Geometry: final body of the model. Coordinates: model frame, mm. Round coordinates to 2 decimals unless told otherwise and drop trailing zeros. Loops run counter-clockwise (first coordinate to the right, second up) from the corner with the lowest first, then second, coordinate; pieces in that order, holes last. Notation, with made-up numbers: (10, -33.75) - (58, -33.75) arc R24 ccw to (58, -8.75) - close; hole circle Ø9 at (11, 2). An arc over 180 degrees is marked (long way). Return JSON: item names as keys, results as strings. Group by question number.
1. Section C-C on y = -11. Return loops of the section in (x, z).
2. Section B-B on y = -6.75. Return loops of the section in (x, z), and give its area (3 significant figures).
3. Section A-A on x = 6. Return loops of the section in (y, z), and give its area (3 significant figures).
4. Material intervals for probe 1 along X at (y, z) = (10.16, 0.25); probe 2 along X at (y, z) = (2.54, 0.2); probe 3 along X at (y, z) = (-7.25, 0.1), sorted ascending.
5. Section D-D on z = 0.1. Count the separate pieces of the cut face and the enclosed holes in it, and give its area (3 significant figures).
from build123d import *

# Parameters (mm, degrees)
BOARD_OUTLINE_START = 0.034
BOARD_OUTLINE_DEPTH = 0.254
SKETCH2_R           = 0.1525
VIA_DEPTH           = 1.288
SKETCH3_R           = 1.397
NPTH_DEPTH          = 1.288
SKETCH4_R           = 0.35
SKETCH4_R_2         = 0.1525
PTH_DEPTH           = 1.288


with BuildPart() as part:
    # Sketch1 → Board_Outline (new body)
    with BuildSketch(Plane.XY.offset(BOARD_OUTLINE_START)):
        with BuildLine():
            ThreePointArc((-8.961, -8.961), (9, -8.961), (9, 9))
            ThreePointArc((9, 9), (-8.961, 9), (-8.961, -8.961))
        make_face()
    extrude(amount=BOARD_OUTLINE_DEPTH)

    # Sketch2 → Via (cut, through all)
    with BuildSketch(Plane.XY):
        with Locations((-1.295, 4.039)):
            Circle(SKETCH2_R)
        with Locations((-3.572, 0.144)):
            Circle(SKETCH2_R)
        with Locations((0.533, 6.325)):
            Circle(SKETCH2_R)
        with Locations((2.896, 5.867)):
            Circle(SKETCH2_R)
        with Locations((1.676, 4.724)):
            Circle(SKETCH2_R)
        with Locations((0.686, -4.115)):
            Circle(SKETCH2_R)
        with Locations((0.838, -5.258)):
            Circle(SKETCH2_R)
        with Locations((0.762, -5.944)):
            Circle(SKETCH2_R)
        with Locations((3.2, -1.295)):
            Circle(SKETCH2_R)
        with Locations((4.496, 2.591)):
            Circle(SKETCH2_R)
        with Locations((3.962, 1.295)):
            Circle(SKETCH2_R)
        with Locations((2.381, -10.211)):
            Circle(SKETCH2_R)
        with Locations((3.429, -2.972)):
            Circle(SKETCH2_R)
        with Locations((1.905, 5.791)):
            Circle(SKETCH2_R)
        with Locations((-3.175, 1.905)):
            Circle(SKETCH2_R)
    extrude(amount=VIA_DEPTH, mode=Mode.SUBTRACT)

    # Sketch3 → NPTH (cut, through all)
    with BuildSketch(Plane.XY):
        with Locations((6.032, -6.032)):
            Circle(SKETCH3_R)
        with Locations((-6.032, 6.032)):
            Circle(SKETCH3_R)
    extrude(amount=NPTH_DEPTH, mode=Mode.SUBTRACT)

    # Sketch4 → PTH (cut, through all)
    with BuildSketch(Plane.XY):
        with Locations((2.286, 9.068)):
            Circle(SKETCH4_R)
        with Locations((1.016, 9.068)):
            Circle(SKETCH4_R)
        with Locations((-0.254, 9.068)):
            Circle(SKETCH4_R)
        with Locations((2.286, 7.798)):
            Circle(SKETCH4_R)
        with Locations((1.016, 7.798)):
            Circle(SKETCH4_R)
        with Locations((-0.254, 7.798)):
            Circle(SKETCH4_R)
        with Locations((-7.62, 2.54)):
            Circle(SKETCH4_R_2)
        with Locations((-7.62, 0)):
            Circle(SKETCH4_R_2)
        with Locations((-10.16, 5.08)):
            Circle(SKETCH4_R_2)
        with Locations((7.62, -2.54)):
            Circle(SKETCH4_R_2)
        with Locations((5.08, 7.62)):
            Circle(SKETCH4_R_2)
        with Locations((-7.62, -7.62)):
            Circle(SKETCH4_R_2)
        with Locations((-5.08, -7.62)):
            Circle(SKETCH4_R_2)
        with Locations((-7.62, -5.08)):
            Circle(SKETCH4_R_2)
        with Locations((-10.16, -2.54)):
            Circle(SKETCH4_R_2)
        with Locations((-10.16, 0)):
            Circle(SKETCH4_R_2)
        with Locations((-10.16, 2.54)):
            Circle(SKETCH4_R_2)
        with Locations((7.62, 2.54)):
            Circle(SKETCH4_R_2)
        with Locations((7.62, 7.62)):
            Circle(SKETCH4_R_2)
        with Locations((-10.16, -5.08)):
            Circle(SKETCH4_R_2)
        with Locations((-5.08, 10.16)):
            Circle(SKETCH4_R_2)
        with Locations((-2.54, 10.16)):
            Circle(SKETCH4_R_2)
    extrude(amount=PTH_DEPTH, mode=Mode.SUBTRACT)


solid = part.part
Taken from the geometry:
{
 "1": {"outline": "(-6.29, 0.03) - (6.33, 0.03) - (6.33, 0.29) - (-6.29, 0.29) - close"},
 "2": {"outline": "(-10.73, 0.03) - (4.83, 0.03) - (4.83, 0.29) - (-10.73, 0.29) - close; (7.23, 0.03) - (10.77, 0.03) - (10.77, 0.29) - (7.23, 0.29) - close", "area": "4.85 mm2"},
 "3": {"outline": "(-11.18, 0.03) - (-7.43, 0.03) - (-7.43, 0.29) - (-11.18, 0.29) - close; (-4.64, 0.03) - (11.22, 0.03) - (11.22, 0.29) - (-4.64, 0.29) - close", "area": "4.98 mm2"},
 "4": {"probe 1": "-7.63 to -5.23, -4.93 to -2.69, -2.39 to 7.67", "probe 2": "-12.43 to -10.31, -10.01 to -7.77, -7.47 to 4.35, 4.64 to 7.47, 7.77 to 12.47", "probe 3": "-10.39 to 5.35, 6.72 to 10.43"},
 "5": {"separate pieces": "1", "enclosed holes": "39", "area": "490 mm2"}
}
